Verification items for this drawing (mm, ordinates from the low corner). A direction names the side the tool comes from. Round coordinates to 2 decimals unless told otherwise and drop trailing zeros. Loops run counter-clockwise (first coordinate to the right, second up) from the corner with the lowest first, then second, coordinate; pieces in that order, holes last. Notation, with made-up numbers: M 52,89 L 60,89 A18 ccw 60,102 Z; hole C 22.25,52.25 d9. An arc over 180 degrees is marked long. Write item = value, one per line. Start each with the question number.
(1) Cross-section at A-A on x = 49. Record the boundary of the cut face in (y, z) (3 decimals), plus the area to 3 significant figures.
(2) Scan lines: L1, parallel to Y at x = 3, z = 14.05 (3 decimals); L2, parallel to Y at x = 29.5, z = 23; L3, parallel to Z at x = 6, y = 9. Record each from-to range of solid material in increasing order. Write a range as from..to.
(3) Go/stop test with flat-tipped pins: P1, Ø0.5, axis at y = 0.5, z = 6, coming from the +X side; P2, Ø8, axis at x = 35.5, z = 19.5, coming from the +Y side; P3, Ø0.8, axis at y = 1.5, z = 1.5, coming from the -X side. Record where each tip stops, or that it passes through.
(4) Cross-section at C-C on x = 3. Record the boundary of the cut face in (y, z) (3 decimals), plus the area to 3 significant figures.
(5) Set-up check for the marked faces 1, 2 and 3: record each of +Z, -Z, +X, -X, +Y, -Y from which the full face is reachable in a straight line by a thin tool's end or side.
(6) Cross-section at B-B on z = 2. Record the boundary of the cut face in (x, y) (3 decimals).
(7) Cross-section at D-D on x = 11. Record the boundary of the cut face in (y, z), plus the area to 3 significant figures.
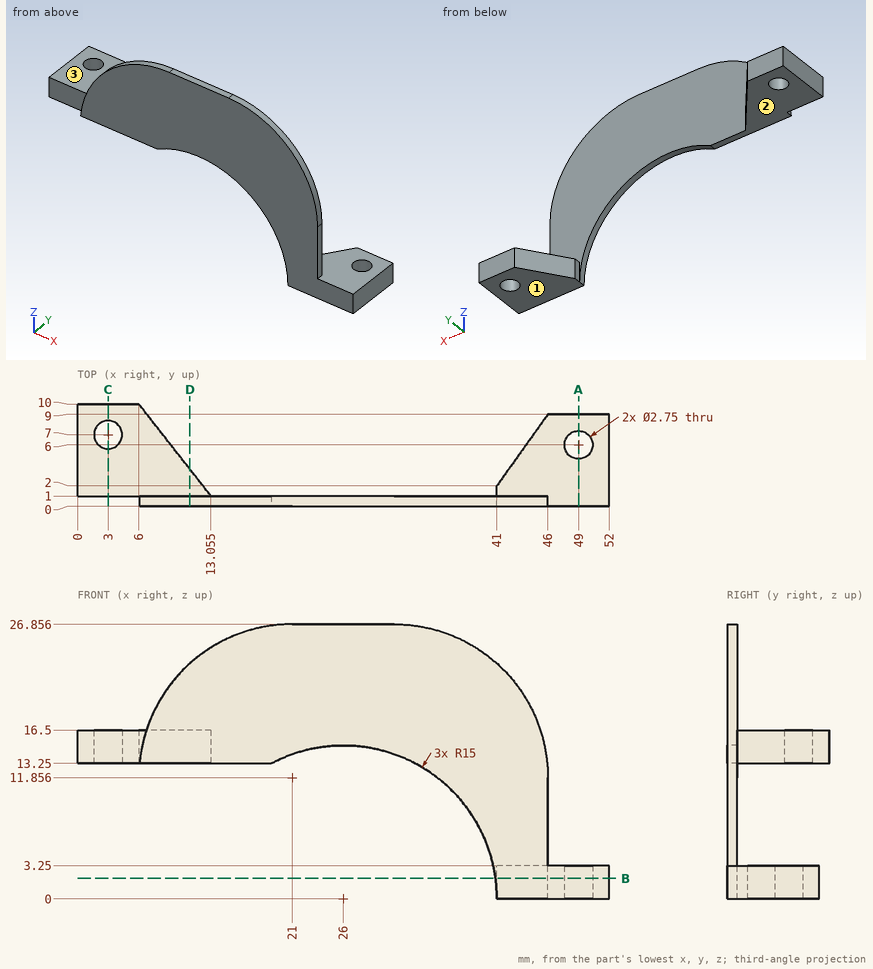
Result:
q1.outline = M 0,0 L 4.625,0 L 4.625,3.25 L 0,3.25 Z; M 7.375,0 L 9,0 L 9,3.25 L 7.375,3.25 Z
q1.area = 20.3 mm^2
q2.L1 = 1..5.625, 8.375..10
q2.L2 = 0..1
q2.L3 = 13.25..16.5
q3.P1 = 46
q3.P2 = 1
q3.P3 = 41
q4.outline = M 1,13.25 L 5.625,13.25 L 5.625,16.5 L 1,16.5 Z; M 8.375,13.25 L 10,13.25 L 10,16.5 L 8.375,16.5 Z
q4.area = 20.3 mm^2
q5.face_1 = -Z, +X, -X, +Y, -Y
q5.face_2 = -Z, -X, +Y, -Y
q5.face_3 = +Z, +X, -X, +Y
q6.outline = M 40.866,0 L 52,0 L 52,9 L 46,9 L 41,2 L 41,1 L 40.866,1 Z; hole C 49,6 d2.75
q7.outline = M 0,13.25 L 3.62,13.25 L 3.62,16.5 L 1,16.5 L 1,23.04 L 0,23.04 Z
q7.area = 18.3 mm^2
